Input: dimensioned drawing with shaded views. Units: mm. Origin: part minimum x, y, z. A direction names the side the tool comes from. Round coordinates to 2 decimals unless told otherwise and drop trailing zeros. Write each loop counter-clockwise with the first axis right and the second up, starting at its lowest first coordinate (ties: lowest second). Pieces come first, ordered by that corner, then holes. Notation, with made-up numbers: (-37.75, -9.75) - (-13.75, -9.75) arc R19 cw to (-13.75, 4.25) - close; hole circle Ø5 at (15, 31). An arc over 180 degrees is marked (long way). Use one line per item in the form item = value.
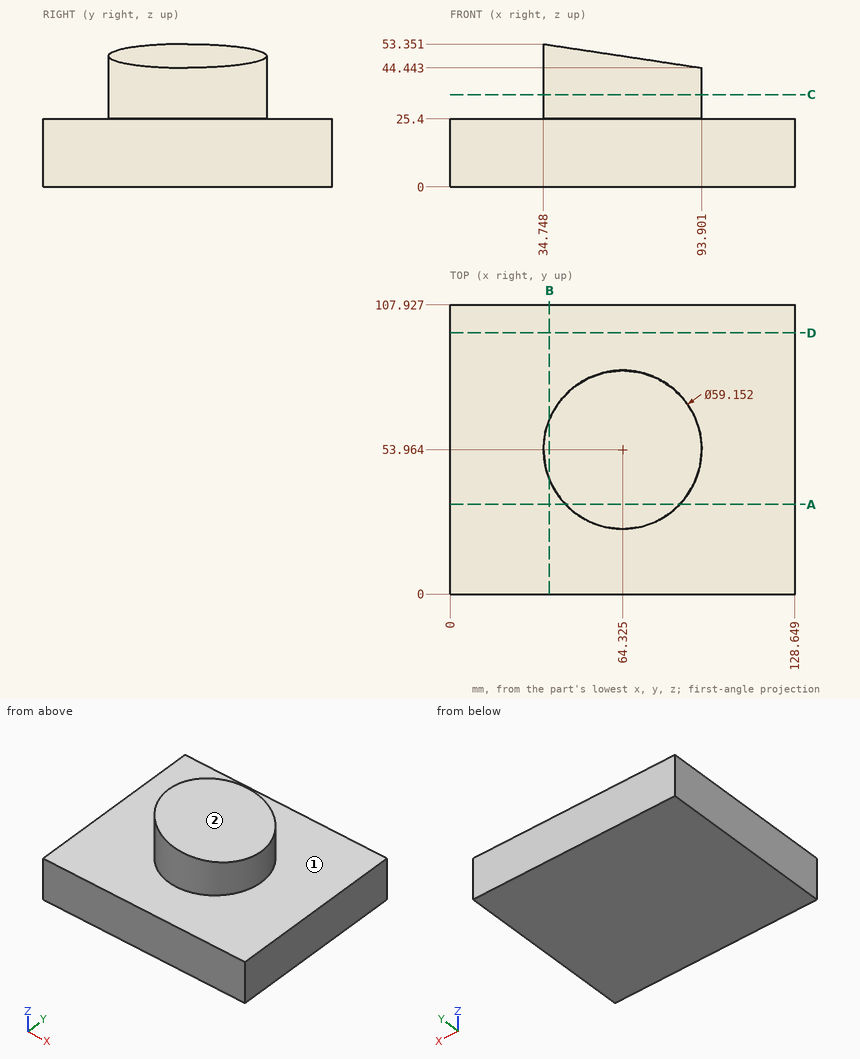
(1) Access query for the marked faces 1 and 2. Directions: +Z, -Z, +X, -X, +Y, -Y. A direction counts if a zero-diameter tool reaches every point of the face in a straight line with its end or side. Return the directions, or none.
Derived:
face_1 = +Z
face_2 = +Z, +X, +Y, -Y
(2) Cut plane B-B on x = 37. Output: boundary loops of the cut face in (y, z) (1 decimal), then the cut area to 3 significant figures.
Derived:
outline = (0, 0) - (107.9, 0) - (107.9, 25.4) - (65.3, 25.4) - (65.3, 53) - (42.6, 53) - (42.6, 25.4) - (0, 25.4) - close
area = 3,370 mm^2
(3) Cut plane C-C on z = 34.5. Output: boundary loops of the cut face in (x, y) (1 decimal), then the cut area to 3 significant figures.
Derived:
outline = circle Ø59.2 at (64.3, 54)
area = 2,750 mm^2
(4) Cut plane D-D on y = 97.5. Output: boundary loops of the cut face in (x, z).
Derived:
outline = (0, 0) - (128.65, 0) - (128.65, 25.4) - (0, 25.4) - close
(5) First-contact query: pin 1 Ø8 at (y, z) = (96.5, 31) entering from -X; pin 2 Ø5 at (x, z) = (79.5, 40.5) entering from +Y (1 decimal); pin 3 Ø10 at (x, y) = (111.5, 28.5) entering from +Z; pin 4 Ø1 at (x, y) = (29, 49) entering from -Z. Flat tips, straight axial feed; report the tip coordinate or a pass-through.
Derived:
pin_1 = through
pin_2 = 80.7
pin_3 = 25.4
pin_4 = 0
(6) Material intervals for L1, parallel to Z at x = 42.5, y = 97; L2, parallel to X at y = 58, z = 32 (1 decimal); L3, parallel to X at y = 41.5, z = 29 (1 decimal), sorted ascending.
Derived:
L1 = 0 to 25.4
L2 = 35 to 93.6
L3 = 37.5 to 91.1
(7) Cut plane A-A on y = 33.5. Output: boundary loops of the cut face in (x, z), then the cut area to 3 significant figures.
Derived:
outline = (0, 0) - (128.65, 0) - (128.65, 25.4) - (85.68, 25.4) - (85.68, 45.68) - (42.97, 52.11) - (42.97, 25.4) - (0, 25.4) - close
area = 4,270 mm^2
